Could you check a few things on this model? Use its own coordinates, in mm. Give positions to 0.01 mm unless a question says otherwise; leave off trailing zeros. Loops run counter-clockwise (first coordinate to the right, second up) from the corner with the lowest first, then second, coordinate; pieces in that order, holes last.
1. Imagine slicing it at A-A (x = 12.5). List the corners of the cut face in (y, z) for me, plus the area to 3 significant figures.
2. For P1, Ø2, axis at x = -1.73, z = 24.82, coming from the +Y side, with a flat end and sliding along its axis, tell me the tip position at first contact or that it passes through.
3. Imagine slicing it at B-B (z = -6). List the corners of the cut face in (x, y) for me.
4. I need wall thicknesses on line 1 along X through (y, z) = (2.4, 12.5); line 2 along Z through (x, y) = (10, 0.7). Which ranges of each line are inside material? Lowest first, please.
5. Imagine slicing it at C-C (y = 1.1). List the corners of the cut face in (x, z) for me, plus the area to 3 significant figures.
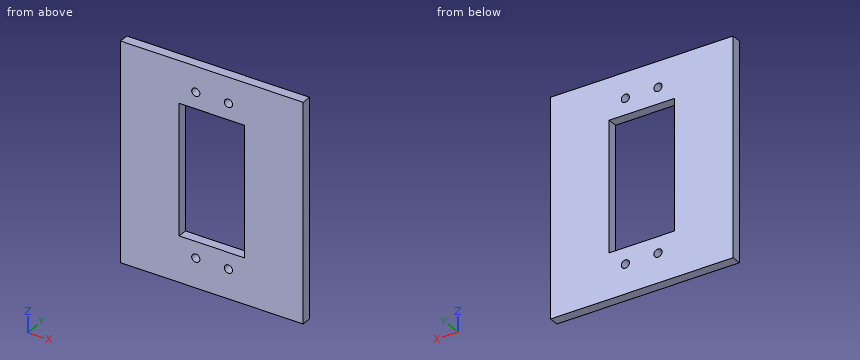
```python
from build123d import *

# Parameters (mm, degrees)
SKETCH1_W           = 55.9
SKETCH1_H           = 66.86
BOSS_EXTRUDE1_DEPTH = 2.95
SKETCH3_W           = 20
SKETCH3_H           = 40
CUT_EXTRUDE1_DEPTH  = 6.86
SKETCH4_R           = 1.25
CUT_EXTRUDE2_DEPTH  = 6.86


with BuildPart() as part:
    # Sketch1 → Boss-Extrude1 (new body)
    with BuildSketch(Plane(origin=(0, 0, 0), x_dir=(1, 0, 0), z_dir=(0, 1, 0))):
        with Locations((3.202267267, 0.752730799)):
            Rectangle(SKETCH1_W, SKETCH1_H)
    extrude(amount=BOSS_EXTRUDE1_DEPTH)

    # Sketch3 → Cut-Extrude1 (cut)
    with BuildSketch(Plane(origin=(0, 2.95, 0), x_dir=(1, 0, 0), z_dir=(0, 1, 0))):
        with Locations((3.202267267, 0.182730799)):
            Rectangle(SKETCH3_W, SKETCH3_H)
    extrude(amount=-CUT_EXTRUDE1_DEPTH, mode=Mode.SUBTRACT)

    # Sketch4 → Cut-Extrude2 (cut)
    with BuildSketch(Plane(origin=(0, 2.95, 0), x_dir=(1, 0, 0), z_dir=(0, 1, 0))):
        with Locations((-1.729576987, 25.182730799)):
            Circle(SKETCH4_R)
        with Locations((8.270423013, 25.182730799)):
            Circle(SKETCH4_R)
        with Locations((-1.729576987, -24.817269201)):
            Circle(SKETCH4_R)
        with Locations((8.270423013, -24.817269201)):
            Circle(SKETCH4_R)
    extrude(amount=-CUT_EXTRUDE2_DEPTH, mode=Mode.SUBTRACT)


solid = part.part
```
Derived:
1. outline: (0, -34.18) - (2.95, -34.18) - (2.95, -20.18) - (0, -20.18) - close; (0, 19.82) - (2.95, 19.82) - (2.95, 32.68) - (0, 32.68) - close
1. area: 79.2 mm2
2. P1: passes through
3. outline: (-24.75, 0) - (-6.8, 0) - (-6.8, 2.95) - (-24.75, 2.95) - close; (13.2, 0) - (31.15, 0) - (31.15, 2.95) - (13.2, 2.95) - close
4. line 1: x = -24.75 to -6.8, 13.2 to 31.15
4. line 2: z = -34.18 to -20.18, 19.82 to 32.68
5. outline: (-24.75, -34.18) - (31.15, -34.18) - (31.15, 32.68) - (-24.75, 32.68) - close; hole (-6.8, -20.18) - (13.2, -20.18) - (13.2, 19.82) - (-6.8, 19.82) - close; hole circle Ø2.5 at (-1.73, -25.18); hole circle Ø2.5 at (-1.73, 24.82); hole circle Ø2.5 at (8.27, -25.18); hole circle Ø2.5 at (8.27, 24.82)
5. area: 2,920 mm2
